Geometry check sheet. Reference: the model listing, model coordinates, mm. Coordinates: 2 decimals unless noted, no trailing zeros. Write each loop counter-clockwise with the first axis right and the second up, starting at its lowest first coordinate (ties: lowest second). Pieces come first, ordered by that corner, then holes. Notation, with made-up numbers: (41.25, 4) -> (91.25, 4) arc R25 ccw to (91.25, 23) -> close; hole circle Ø2 at (4.5, 3.5). An arc over 180 degrees is marked (long way). Answer in a Markdown table with one row per item. Add a question column.
1. Mould release check, pull along Y, two halves, no side actions. Record for faces 1 (the cylindrical face through (1.93, -1.341, 3.233)), 2 (the cylindrical face through (0.838, 0.33, 7.493)), 3 (the flat face through (-7, 0, 0)): pulls with the +Y half, pulls with the -Y half, needs draft (parallel to the pull), parting line crosses it, or undercut.
2. Scan lines: L1, parallel to Y at x = 3, z = 0; L2, parallel to Y at x = -1.75, z = -2.5; L3, parallel to Z at x = -3.5, y = 0.25. Record each from-to range of solid material in increasing order. Write a range as from..to.
3. Depth check by flat-ended pin: P1, Ø5, axis at x = 1.5, z = 3.5, coming from the +Y side; P2, Ø5, axis at x = -1.5, y = -5.5, coming from the -Z side; P3, Ø4, axis at y = -1, z = 0.5, coming from the +X side. Enter the tip coordinate at first touch or a pass-through.
4. Cross-section at A-A on x = 1. Record the cut outline in (y, z), and give its area (3 significant figures).
```python
from build123d import *

# Parameters (mm, degrees)
SKETCH1_R                 = 7.5
BOSS_EXTRUDE1_DEPTH       = 7
M8X1_0_TAPPED_HOLE1_D     = 7
M8X1_0_TAPPED_HOLE1_DEPTH = 10
M8X1_0_TAPPED_HOLE1_TIP   = 2.103012167
FILLET1_R                 = 1.5


with BuildPart() as part:
    # Sketch1 → Boss-Extrude1 (new, symmetric)
    with BuildSketch(Plane(origin=(0, 0, 0), x_dir=(0, 0, -1), z_dir=(1, 0, 0))):
        Circle(SKETCH1_R)
    extrude(amount=BOSS_EXTRUDE1_DEPTH, both=True)

    # M8x1.0 Tapped Hole1
    with Locations(Plane(origin=(7, 0, 0), x_dir=(0, 0, -1), z_dir=(1, 0, 0))):
        with Locations((0, 0)):
            Hole(M8X1_0_TAPPED_HOLE1_D / 2, depth=M8X1_0_TAPPED_HOLE1_DEPTH)
            with Locations((0, 0, -(M8X1_0_TAPPED_HOLE1_DEPTH + M8X1_0_TAPPED_HOLE1_TIP / 2))):  # 118° drill point
                Cone(0, M8X1_0_TAPPED_HOLE1_D / 2, M8X1_0_TAPPED_HOLE1_TIP, mode=Mode.SUBTRACT)

    # Fillet1
    fillet1_edges = [part.edges().sort_by_distance(p)[0] for p in [
        (-7, 0, 7.5),
    ]]
    fillet(fillet1_edges, radius=FILLET1_R)


solid = part.part
```
Results found:
| question | item | result |
|---|---|---|
| 1 | face 1 | undercut |
| 1 | face 2 | parting line crosses it |
| 1 | face 3 | needs draft |
| 2 | L1 | y = -7.5..-3.5, 3.5..7.5 |
| 2 | L2 | y = -7.07..-2.45, 2.45..7.07 |
| 2 | L3 | z = -7.5..-2.66, 2.66..7.5 |
| 3 | P1 | stops at y = 7.43 |
| 3 | P2 | stops at z = -6.87 |
| 3 | P3 | stops at x = -3.23 |
| 4 | outline | circle Ø15 at (0, 0); hole circle Ø7 at (0, 0) |
| 4 | area | 138 mm^2 |
